from build123d import *

# Parameters (mm, degrees)
F0_W     = 31.46597
F0_H     = 31.925406
F1_DEPTH = 1
F2_R     = 2.098305
F3_DEPTH = 31.925406
F4_W     = 12.19663
F4_H     = 22.610463
F5_DEPTH = 3.81


with BuildPart() as f1:
    # F0 (on Front) → F1 (new body)
    with BuildSketch(Plane.XZ):
        with Locations((15.732985, 15.962703)):
            Rectangle(F0_W, F0_H)
    extrude(amount=F1_DEPTH)

    # F2 (on face) → F3 (join, through all)
    with BuildSketch(Plane.XY.offset(31.925406)):
        with BuildLine():
            Line((31.46597, -1), (31.655797, -1.462564))
            ThreePointArc((31.655797, -1.462564), (36.536716, -0.5), (31.655797, 0.462564))
            Line((31.655797, 0.462564), (31.46597, 0))
            Line((31.46597, 0), (31.46597, -1))
        make_face()
        with Locations((34.001343, -0.5)):
            Circle(F2_R, mode=Mode.SUBTRACT)
    extrude(amount=-F3_DEPTH)

    # F4 (on face) → F5 (cut, symmetric)
    with BuildSketch(Plane.XZ.offset(1)):
        with Locations((31.46597, 15.962703)):
            Rectangle(F4_W, F4_H)
    extrude(amount=F5_DEPTH, both=True, mode=Mode.SUBTRACT)


solid = f1.part
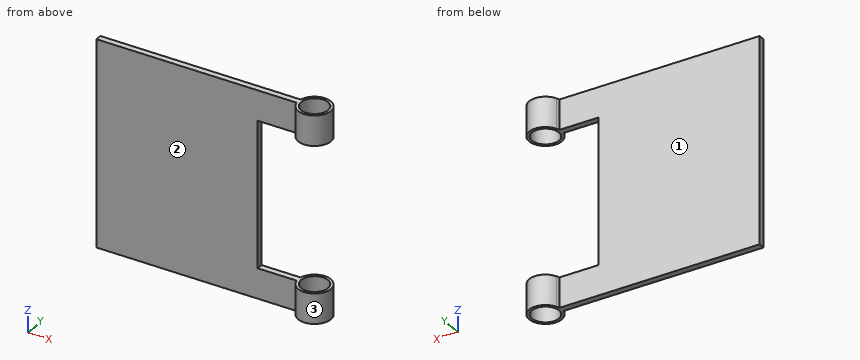
Here's how the part is built. I have some questions about the finished solid (model axes, mm). Face numbers are marked on the shaded views. A direction names the side the tool comes from. Coordinates: 2 decimals unless noted, no trailing zeros. Write each loop counter-clockwise with the first axis right and the second up, starting at its lowest first coordinate (ties: lowest second). Pieces come first, ordered by that corner, then holes.
Item 1: I want a section at C-C on z = 15. Write out the boundary of the cut face in (x, y).
Item 2: I want a section at A-A on x = 31. Write out the boundary of the cut face in (y, z).
Item 3: On a 3-axis mill with a long thin cutter (end or side, diameter ignored), from which of +Z, -Z, +X, -X, +Y, -Y can I reach the whole of each face in a straight line? I mean the marked faces 1, 2 and 3. Say none if no direction works.
Item 4: Will these pins go through, and if not, where does the flat tip stop? pin 1 (15.5 mm diameter, centred on x = 15.5, z = 12, fed in from -Y); pin 2 (1.5 mm diameter, centred on x = 15.5, z = 22.5, fed in from +Y); pin 3 (0.5 mm diameter, centred on y = -0.5, z = 11.5, fed in from +X).
Item 5: I want a section at B-B on y = -0.5. Write out the boundary of the cut face in (x, z).
Item 6: I want a section at D-D on x = 3. Write out the boundary of the cut face in (y, z), and give its area (3 significant figures).
Item 7: If I drill on line 1 (Z direction, x = 26, y = -0.95); line 2 (Y direction, x = 14, z = 13); line 3 (X direction, y = -0.75, z = 19.5), over which ranges is the centre line in solid material (lowest first)?
Findings below:
1. outline: (0, -1) - (25.37, -1) - (25.37, 0) - (0, 0) - close
2. outline: (-1, 0) - (0, 0) - (0, 4.66) - (-1, 4.66) - close; (-1, 27.27) - (0, 27.27) - (0, 31.93) - (-1, 31.93) - close
3. face 1: +Z, -Z, -X, +Y
3. face 2: +Z, -Z, -X, -Y
3. face 3: +Z, -Z
4. pin 1: stops at y = -1
4. pin 2: stops at y = 0
4. pin 3: stops at x = 25.37
5. outline: (0, 0) - (31.9, 0) - (31.9, 4.66) - (25.37, 4.66) - (25.37, 27.27) - (31.9, 27.27) - (31.9, 31.93) - (0, 31.93) - close; (36.1, 0) - (36.54, 0) - (36.54, 4.66) - (36.1, 4.66) - close; (36.1, 27.27) - (36.54, 27.27) - (36.54, 31.93) - (36.1, 31.93) - close
6. outline: (-1, 0) - (0, 0) - (0, 31.93) - (-1, 31.93) - close
6. area: 31.9 mm2
7. line 1: z = 0 to 4.66, 27.27 to 31.93
7. line 2: y = -1 to 0
7. line 3: x = 0 to 25.37
